```python
from build123d import *

# Parameters (mm, degrees)
BOSS_EXTRUDE1_DEPTH                               = 20
SKETCH2_R                                         = 6.25
SKETCH2_R_2                                       = 7.5
CUT_EXTRUDE1_DEPTH                                = 141.445719052
SKETCH3_R                                         = 10
SKETCH3_W                                         = 80
SKETCH3_H                                         = 15
CUT_EXTRUDE3_DEPTH                                = 137.106575888
CSK_FOR_M3_5_FLAT_HEAD_MACHINE_SCREW1_D           = 3.9
CSK_FOR_M3_5_FLAT_HEAD_MACHINE_SCREW1_CSINK_D     = 8.2
CSK_FOR_M3_5_FLAT_HEAD_MACHINE_SCREW1_CSINK_ANGLE = 90
FILLET2_R                                         = 7.5
FILLET4_R                                         = 5
FILLET2_OF_MIRROR2_R                              = 7.5
FILLET4_OF_MIRROR2_R                              = 5


with BuildPart() as part:
    # Sketch1 → Boss-Extrude1 (new, symmetric)
    with BuildSketch(Plane.XY):
        with BuildLine():
            Line((0, -50), (-125, -50))
            Line((-125, -50), (-125, -29.356175837))
            ThreePointArc((-125, -29.356175837), (-77.109944012, -7.490693948), (-25, 0))
            Line((-25, 0), (0, 0))
            Line((0, 0), (0, -50))
        make_face()
    boss_extrude1 = extrude(amount=BOSS_EXTRUDE1_DEPTH, both=True)

    # Sketch2 → Cut-Extrude1 (cut, through all)
    with BuildSketch(Plane.XY.offset(20)):
        with Locations((-105, -35)):
            Circle(SKETCH2_R)
        with Locations((-65, -27.5)):
            Circle(SKETCH2_R_2)
    cut_extrude1 = extrude(amount=-CUT_EXTRUDE1_DEPTH, mode=Mode.SUBTRACT)

    # Sketch3 → Cut-Extrude3 (cut, through all)
    with BuildSketch(Plane(origin=(0, -50, 0), x_dir=(-1, 0, 0), z_dir=(0, -1, 0))):
        with Locations((45, 0)):
            Circle(SKETCH3_R)
        with Locations((85, 0)):
            Rectangle(SKETCH3_W, SKETCH3_H)
    cut_extrude3 = extrude(amount=-CUT_EXTRUDE3_DEPTH, mode=Mode.SUBTRACT)

    # CSK for M3.5 Flat Head Machine Screw1 (through all)
    with Locations(Plane(origin=(0, 0, 0), x_dir=(1, 0, 0), z_dir=(0, 1, 0))):
        with Locations((-12.5, 0)):
            csk_for_m3_5_flat_head_machine_screw1 = CounterSinkHole(CSK_FOR_M3_5_FLAT_HEAD_MACHINE_SCREW1_D / 2, CSK_FOR_M3_5_FLAT_HEAD_MACHINE_SCREW1_CSINK_D / 2, counter_sink_angle=CSK_FOR_M3_5_FLAT_HEAD_MACHINE_SCREW1_CSINK_ANGLE)

    # Fillet2
    fillet2_edges = [part.edges().sort_by_distance(p)[0] for p in [
        (-125, -50, -13.75),
        (-125, -29.356175837, -13.75),
        (-125, -50, 13.75),
        (-125, -29.356175837, 13.75),
    ]]
    fillet(fillet2_edges, radius=FILLET2_R)

    # Fillet4
    fillet4_edges = [part.edges().sort_by_distance(p)[0] for p in [
        (-51.614378278, -25.96220061, 7.5),
        (-51.614378278, -25.96220061, -7.5),
    ]]
    fillet(fillet4_edges, radius=FILLET4_R)

    # Mirror2: Boss-Extrude1, Cut-Extrude1, Cut-Extrude3, CSK for M3.5 Flat Head Machine Screw1 across plane
    add(boss_extrude1.mirror(Plane(origin=(0, 0, 20), x_dir=(0, 0, 1), z_dir=(-1, 0, 0))))
    add(cut_extrude1.mirror(Plane(origin=(0, 0, 20), x_dir=(0, 0, 1), z_dir=(-1, 0, 0))), mode=Mode.SUBTRACT)
    add(cut_extrude3.mirror(Plane(origin=(0, 0, 20), x_dir=(0, 0, 1), z_dir=(-1, 0, 0))), mode=Mode.SUBTRACT)
    add(csk_for_m3_5_flat_head_machine_screw1.mirror(Plane(origin=(0, 0, 20), x_dir=(0, 0, 1), z_dir=(-1, 0, 0))), mode=Mode.SUBTRACT)

    # Fillet2 of Mirror2
    fillet2_of_mirror2_edges = [part.edges().sort_by_distance(p)[0] for p in [
        (125, -50, -13.75),
        (125, -29.356175837, -13.75),
        (125, -50, 13.75),
        (125, -29.356175837, 13.75),
    ]]
    fillet(fillet2_of_mirror2_edges, radius=FILLET2_OF_MIRROR2_R)

    # Fillet4 of Mirror2
    fillet4_of_mirror2_edges = [part.edges().sort_by_distance(p)[0] for p in [
        (51.614378278, -25.96220061, 7.5),
        (51.614378278, -25.96220061, -7.5),
    ]]
    fillet(fillet4_of_mirror2_edges, radius=FILLET4_OF_MIRROR2_R)


solid = part.part
```
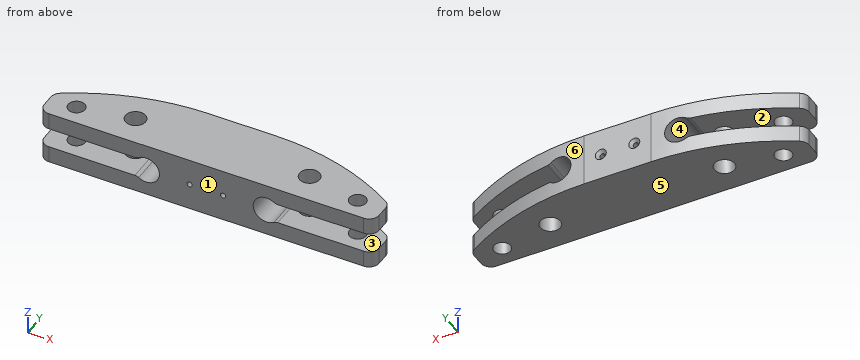
Geometry: final body of the model. Coordinates: model frame, mm. Face numbers are marked on the shaded views. A direction names the side the tool comes from. Coordinates: 2 decimals unless noted, no trailing zeros. Order: outer loops, then holes, each group sorted by start corner. A loop starts at its lowest first (then second) coordinate and runs counter-clockwise, first axis right, second up. Notation, with made-up numbers: (-9.75, 48) - (41.25, 48) arc R25 cw to (41.25, 74) - close; hole circle Ø2 at (32, -38). An arc over 180 degrees is marked (long way). Write each question's results on one line, items separated by ' | '.
(1) Section query A-A, the plane x = -65. Return the cut outline in (y, z).
Values found:
outline: (-50, -20) - (-35, -20) - (-35, -7.5) - (-50, -7.5) - close; (-50, 7.5) - (-35, 7.5) - (-35, 20) - (-50, 20) - close; (-20, -20) - (-4.38, -20) - (-4.38, -7.5) - (-20, -7.5) - close; (-20, 7.5) - (-4.38, 7.5) - (-4.38, 20) - (-20, 20) - close
(2) Line query: line 1 (X direction, y = -22, z = 15.5); line 2 (Z direction, x = 61, y = -45.5); line 3 (Z direction, x = 12.5, y = -27). Output: solid intervals per line, ascending. Write a range as [from, to].
Values found:
line 1: x = [-112.5, -70.1], [-59.9, 59.9], [70.1, 112.5] | line 2: z = [-20, -7.5], [7.5, 20] | line 3: z = [-20, -1.95], [1.95, 20]
(3) First-contact query: pin 1 Ø9 at (x, y) = (65, -27.5) entering from -Z; pin 2 Ø1 at (y, z) = (-26, -3.5) entering from -X; pin 3 Ø4 at (y, z) = (-29, 13.5) entering from +X; pin 4 Ø5 at (x, z) = (12.5, 0) entering from +Y. Flat tips, straight axial feed; report the tip coordinate or a pass-through.
Values found:
pin 1: passes through | pin 2: stops at x = -35.83 | pin 3: stops at x = 124.57 | pin 4: stops at y = -1.6
(4) Section query C-C, the plane y = -6. Return the cut outline in (x, z), plus the area to 3 significant figures.
Values found:
outline: (-71.73, -20) - (71.73, -20) - (71.73, -7.5) - (53.29, -7.5) arc R5 ccw to (50.53, -8.33) arc R10 cw (long way) to (50.53, 8.33) arc R5 ccw to (53.29, 7.5) - (71.73, 7.5) - (71.73, 20) - (-71.73, 20) - (-71.73, 7.5) - (-53.29, 7.5) arc R5 ccw to (-50.53, 8.33) arc R10 cw (long way) to (-50.53, -8.33) arc R5 ccw to (-53.29, -7.5) - (-71.73, -7.5) - close; hole circle Ø3.9 at (-12.5, 0); hole circle Ø3.9 at (12.5, 0) | area: 4,550 mm²
(5) Section query D-D, the plane x = -39. Return the cut outline in (y, z).
Values found:
outline: (-50, -20) - (-0.53, -20) - (-0.53, -8) - (-50, -8) - close; (-50, 8) - (-0.53, 8) - (-0.53, 20) - (-50, 20) - close
(6) Set-up query: the marked faces 1, 2 and 3. Return all of +Z, -Z, +X, -X, +Y, -Y with unobstructed straight access to the full face (end or side cutting, diameter ignored); none if empty.
Values found:
face 1: +Z, -Z, +X, -X, -Y | face 2: -X, +Y, -Y | face 3: +X, +Y, -Y
(7) Mould query, pull axis X, two halves, no side actions, for the marked faces 4, 5 and 6. Classes: +X half, -X half, draft (parallel to the pull), parting line (faces both ways), or undercut.
Values found:
face 4: undercut | face 5: draft | face 6: +X half
(8) Section query B-B, the plane z = -16.5. Return the cut outline in (x, y).
Values found:
outline: (-125, -42.5) arc R7.5 ccw to (-117.5, -50) - (117.5, -50) arc R7.5 ccw to (125, -42.5) - (125, -33.51) arc R7.5 ccw to (121.41, -27.11) arc R185 ccw to (25, 0) - (-25, 0) arc R185 ccw to (-121.41, -27.11) arc R7.5 ccw to (-125, -33.51) - close; hole circle Ø12.5 at (-105, -35); hole circle Ø15 at (-65, -27.5); hole circle Ø15 at (65, -27.5); hole circle Ø12.5 at (105, -35)
